Autodesk Inventor part; units mm, degrees
ref_plane "YZ Plane" through (0, 0, 0) normal (1, 0, 0) x (0, 1, 0)
ref_plane "XZ Plane" through (0, 0, 0) normal (0, 1, 0) x (-1, 0, 0)
ref_plane "XY Plane" through (0, 0, 0) normal (0, 0, 1) x (1, 0, 0)
sketch "Sketch1" plane through (0, 0, 0) normal (0, 1, 0) x (-1, 0, 0)
  line L0 (-10, 17.5) -> (10, 17.5)
  line L1 (10, 17.5) -> (10, -17.5)
  line L2 (10, -17.5) -> (-10, -17.5)
  line L3 (-10, -17.5) -> (-10, 17.5)
  line L4 (-10, 17.5) -> (10, -17.5) construction
  line L5 (10, 17.5) -> (-10, -17.5) construction
  point P0 (0, 0)
  dimension "d0" = 35
  dimension "d1" = 20
extrude "Extrusion1" add sketch "Sketch1" along normal blind 140
sketch "Sketch2" plane through (0, 140, 0) normal (0, 1, 0) x (1, 0, 0)
  line L0 (-10, 27.5) -> (-10, -27.5)
  line L1 (-10, -27.5) -> (-20, -27.5)
  line L2 (-10, 27.5) -> (-20, 27.5)
  line L3 (-20, 27.5) -> (-20, -27.5)
  line L4 (-10, 17.5) -> (-10, -17.5)
  point P0 (0, 0)
  dimension "d4" = 55
  dimension "d5" = 0
  dimension "d6" = 10
  dimension "d7" = 27.5
extrude "Extrusion2" add sketch "Sketch2" against normal blind 140
sketch "Sketch3" plane through (0, 140, 0) normal (0, 1, 0) x (1, 0, 0)
  line L0 (10, -17.5) -> (10, 17.5)
  point P0 (0, 0)
  point P1 (3, -10.5)
  dimension "d10" = 7
  dimension "d11" = 10.5
hole "Hole1" at (3, 140, 10.5) direction (0, -1, 0) diameter 4.917 depth 20 tip angle 118
pattern_linear "Rectangular Pattern1" count 2 spacing 16 along (-1, 0, 0) count 2 spacing 21 along (0, 0, -1) of "Hole1"
sketch "Sketch4" plane through (0, 0, 0) normal (0, -1, 0) x (1, 0, 0)
  line L0 (10, 17.5) -> (10, -17.5)
  point P0 (0, 0)
  point P1 (-13, -10.5)
  point P2 (-13, 10.5)
  point P3 (2, 0)
  dimension "d25" = 21
  dimension "d27" = 10.5
  dimension "d28" = 23
  dimension "d29" = 23
  dimension "d30" = 8
  dimension "d31" = 15
hole "Hole2" at (-13, 0, -10.5) at (-13, 0, 10.5) at (2, 0, 0) direction (0, 1, 0) diameter 6.647 depth 20 tip angle 118
sketch "Sketch5" plane through (10, 0, 17.5) normal (1, 0, 0) x (0, 0, -1)
  line L0 (0, 0) -> (35, 0)
  point P0 (17.5, 0)
  point P1 (30, 25)
  point P2 (17.5, 0)
  point P3 (17.5, 0)
  dimension "d39" = 25
  dimension "d40" = 12.5
hole "Hole3" at (10, 25, -12.5) direction (-1, 0, 0) diameter 4.917 depth 15 tip angle 118
pattern_linear "Rectangular Pattern2" count 2 spacing 25 along (0, 0, 1) count 3 spacing 45 along (0, 1, 0) of "Hole3"
properties part number "Fuhrung"
Verification items for the finished model (mm, model axes). A direction names the side the tool comes from. Coordinates: 2 decimals unless noted, no trailing zeros. Loops run counter-clockwise (first coordinate to the right, second up) from the corner with the lowest first, then second, coordinate; pieces in that order, holes last. Notation, with made-up numbers: (85, 39.25) - (120, 39.25) arc R27 cw to (120, 55.25) - close; hole circle Ø6 at (52, 39.5). An arc over 180 degrees is marked (long way). Answer as a JSON object with one key per item and string values.
(1) Access from +Z, -Z, +X, -X, +Y, -Y to the whole of each face (thin tool, end or side, straight path). Record for faces 5 (the cylindrical face through (2.39, 26.5, -10.55)), 6 (the cylindrical face through (-15.438, 129.86, 10.18)), 7 (the flat face through (0, 69, -17.5)), 8 (the conical face through (-12.97, 21.65, 11.08)), 9 (the flat face through (10, 69, 0)).
Response:
{"face 5": "+X", "face 6": "+Y", "face 7": "-Z, +X, +Y, -Y", "face 8": "-Y", "face 9": "+Z, -Z, +X, +Y, -Y"}
(2) Scan lines: line 1 along Y through (x, z) = (-1.5, 12.5); line 2 along Z through (x, y) = (1, 115); line 3 along X through (y, z) = (134.5, 10.5). Record each from-to range of solid material in increasing order.
Response:
{"line 1": "y = 0 to 22.54, 27.46 to 67.54, 72.46 to 112.54, 117.46 to 140", "line 2": "z = -17.5 to -14.96, -10.04 to 10.04, 14.96 to 17.5", "line 3": "x = -20 to -15.46, -10.54 to 0.54, 5.46 to 10"}
(3) Go/stop test with flat-tipped pins: pin 1 Ø16 at (x, y) = (-1, 94) entering from -Z; pin 2 Ø11 at (y, z) = (40.5, 25) entering from +X; pin 3 Ø4 at (x, z) = (2, 0) entering from -Y; pin 4 Ø8 at (x, z) = (-13, -10.5) entering from -Y. Record where each tip stops, or that it passes through.
Response:
{"pin 1": "stops at z = -17.5", "pin 2": "stops at x = -10", "pin 3": "stops at y = 20.8", "pin 4": "stops at y = 0"}
(4) Cross-section at A-A, the plane y = 34. Record the boundary of the cut face in (x, z).
Response:
{"outline": "(-20, -27.5) - (-10, -27.5) - (-10, -17.5) - (10, -17.5) - (10, 17.5) - (-10, 17.5) - (-10, 27.5) - (-20, 27.5) - close"}
(5) Mould release check, pull along Y, two halves, no side actions. Record for faces 1 (the flat face through (-8, 0, 0)), 2 (the flat face through (-20, 71, 0)), 3 (the flat face through (-8, 140, 0)), 4 (the conical face through (-6.22, 24.58, 12.59)): pulls with the +Y half, pulls with the -Y half, needs draft (parallel to the pull), parting line crosses it, or undercut.
Response:
{"face 1": "pulls with the -Y half", "face 2": "needs draft", "face 3": "pulls with the +Y half", "face 4": "undercut"}
